The listing builds one solid part. Answer for the finished solid, in the listing's coordinates (mm). Give positions to 0.01 mm unless a question says otherwise; leave off trailing zeros. Order: outer loops, then holes, each group sorted by start corner. A loop starts at its lowest first (then second) coordinate and runs counter-clockwise, first axis right, second up. Notation, with made-up numbers: (-20, -4.5) - (14, -4.5) arc R22 cw to (14, 32.5) - close; hole circle Ø9 at (-20, 50). An arc over 180 degrees is marked (long way). Write each question's results on one line, items separated by ' | '. Start each with the question number.
1. Find the intervals of material crossed by L1, parallel to Z at x = -31.5, y = -12, in increasing order.
2. Section B-B (y = 10) is taken. Give the vertices of the cut face in (x, z).
3. Flat-ended cylindrical pins translate along their axes: pin 1 (2 mm diameter, centred on x = -27, y = -22.5, fed in from +Z); pin 2 (10 mm diameter, centred on x = 18.5, y = 4, fed in from -Z). Find the tip coordinate at first contact, or state that the pin passes through.
4. Determine the mould class of faces 1 (the face through (-1, 3, 2.9)), 2 (the face through (-1, -33.6, 1)), 3 (the face through (-52.75, 0, 1)) for opening direction Y: released by +Y, released by -Y, zero draft, split by the parting line, or undercut.
5. Section A-A (x = 35) is taken. Give the vertices of the cut face in (y, z).
from build123d import *

# Parameters (mm, degrees)
SKETCH1_W           = 105.5
SKETCH1_H           = 67.2
SKETCH1_W_2         = 98.9
SKETCH1_H_2         = 57.7
BOSS_EXTRUDE1_DEPTH = 3
SKETCH1_3_W         = 98.9
SKETCH1_3_H         = 57.7
SKETCH1_3_W_2       = 95.04
SKETCH1_3_H_2       = 53.856
BOSS_EXTRUDE2_DEPTH = 2.95
SKETCH1_4_W         = 95.04
SKETCH1_4_H         = 53.856
BOSS_EXTRUDE3_DEPTH = 2.9


with BuildPart() as part:
    # Sketch1 → Boss-Extrude1 (new body)
    with BuildSketch(Plane.XY):
        Rectangle(SKETCH1_W, SKETCH1_H)
        with Locations((0, 2.45)):
            Rectangle(SKETCH1_W_2, SKETCH1_H_2, mode=Mode.SUBTRACT)
    extrude(amount=BOSS_EXTRUDE1_DEPTH)

    # Sketch1<3> → Boss-Extrude2 (add)
    with BuildSketch(Plane.XY):
        with Locations((0, 2.45)):
            Rectangle(SKETCH1_3_W, SKETCH1_3_H)
        with Locations((0, 2.452)):
            Rectangle(SKETCH1_3_W_2, SKETCH1_3_H_2, mode=Mode.SUBTRACT)
    extrude(amount=BOSS_EXTRUDE2_DEPTH)

    # Sketch1<4> → Boss-Extrude3 (add)
    with BuildSketch(Plane.XY):
        with Locations((0, 2.452)):
            Rectangle(SKETCH1_4_W, SKETCH1_4_H)
    extrude(amount=BOSS_EXTRUDE3_DEPTH)


solid = part.part
Reported:
1) L1: 0 to 2.9
2) outline: (-52.75, 0) - (52.75, 0) - (52.75, 3) - (49.45, 3) - (49.45, 2.95) - (47.52, 2.95) - (47.52, 2.9) - (-47.52, 2.9) - (-47.52, 2.95) - (-49.45, 2.95) - (-49.45, 3) - (-52.75, 3) - close
3) pin 1: z = 2.9 | pin 2: z = 0
4) face 1: undercut | face 2: released by -Y | face 3: zero draft
5) outline: (-33.6, 0) - (33.6, 0) - (33.6, 3) - (31.3, 3) - (31.3, 2.95) - (29.38, 2.95) - (29.38, 2.9) - (-24.48, 2.9) - (-24.48, 2.95) - (-26.4, 2.95) - (-26.4, 3) - (-33.6, 3) - close
